```python
from build123d import *

# Parameters (mm, degrees)
F0_W     = 1450
F0_H     = 100
F4_DEPTH = 50
F1_SIZE  = 49.99999
F2_SIZE  = 49.99999
F3_R     = 5


# Not quite as in the source:
# - a fillet or chamfer is up to 0.001 mm smaller than in the source, because OpenCascade refuses the exact size


with BuildPart() as f4:
    # F0 (on Front) → F4 (new body)
    with BuildSketch(Plane.XZ):
        with Locations((74.6626051481, 50)):
            Rectangle(F0_W, F0_H)
    extrude(amount=F4_DEPTH)

    # F1 (size 50 in the source; OpenCascade refuses exactly that, so slightly less here)
    f1_edges = [f4.edges().sort_by_distance(p)[0] for p in [
        (799.662605, -50, 50),
    ]]
    chamfer(f1_edges, length=F1_SIZE)

    # F2 (size 50 in the source; OpenCascade refuses exactly that, so slightly less here)
    f2_edges = [f4.edges().sort_by_distance(p)[0] for p in [
        (-650.337395, -50, 50),
    ]]
    chamfer(f2_edges, length=F2_SIZE)

    # F3
    f3_edges = [f4.edges().sort_by_distance(p)[0] for p in [
        (74.662605, -50, 100),
        (74.662605, -50, 0),
        (74.662605, 0, 100),
        (74.662605, 0, 0),
    ]]
    fillet(f3_edges, radius=F3_R)


solid = f4.part
```
Geometry: final body of the model. Coordinates: model frame, mm. Round coordinates to 2 decimals unless told otherwise and drop trailing zeros. Write each loop counter-clockwise with the first axis right and the second up, starting at its lowest first coordinate (ties: lowest second). Pieces come first, ordered by that corner, then holes. Notation, with made-up numbers: (47, 42) -> (53, 42) arc R15 cw to (53, 71) -> close; hole circle Ø5 at (50, -5). An arc over 180 degrees is marked (long way). Return JSON: item names as keys, results as strings.
Q1. Section B-B on y = -14. Return the cut outline in (x, z).
From the geometry:
{"outline": "(-636.34, 0) -> (785.66, 0) -> (785.66, 100) -> (-636.34, 100) -> close"}
Q2. First-contact query: pin 1 Ø5 at (y, z) = (-13, 78.5) entering from -X; pin 2 Ø8 at (y, z) = (-6, 50) entering from +X; pin 3 Ø8 at (y, z) = (-43.5, 31.5) entering from -X. Flat tips, straight axial feed; report the tip coordinate or a pass-through.
From the geometry:
{"pin 1": "x = -639.84", "pin 2": "x = 797.66", "pin 3": "x = -610.84"}
Q3. Ray query, line 1 (Z direction, x = 199.5, y = -46); line 2 (Z direction, x = 272.5, y = -46.5); line 3 (X direction, y = -47, z = 13). Return the intervals inside material, ascending.
From the geometry:
{"line 1": "0.1 to 99.9", "line 2": "0.23 to 99.77", "line 3": "-603.34 to 752.66"}
